Autodesk Inventor part; units mm, degrees
ref_plane "YZ Plane" through (0, 0, 0) normal (1, 0, 0) x (0, 1, 0)
ref_plane "XZ Plane" through (0, 0, 0) normal (0, 1, 0) x (-1, 0, 0)
ref_plane "XY Plane" through (0, 0, 0) normal (0, 0, 1) x (1, 0, 0)
sketch "Sketch1" plane through (0, 0, 0) normal (0, 0, 1) x (1, 0, 0)
  arc A0 (25.4, 0) -> (-25.4, 0.0312) centre (0, 0) ccw
  arc A1 (31.75, 0) -> (-31.75, 0.039) centre (0, 0) ccw
  arc A2 (-31.75, 0.039) -> (-25.4, 0.0312) centre (-28.575, 0.0351) ccw
  line L0 (25.4, 0) -> (25.4, -50.8)
  line L1 (25.4, -50.8) -> (31.75, -50.8)
  line L2 (31.75, -50.8) -> (31.75, 0)
  line L3 (25.4, 0) -> (31.75, 0) construction
  dimension "d0" = 6.35
  dimension "d1" = 25.4
  dimension "d2" = 50.8
extrude "Extrusion1" add sketch "Sketch1" along normal blind 6.35
properties part number "HangHook" material "Steel, High Strength Low Alloy"
Geometry: final body of the model. Coordinates: model frame, mm. Give positions to 0.01 mm unless a question says otherwise; leave off trailing zeros. Loops run counter-clockwise (first coordinate to the right, second up) from the corner with the lowest first, then second, coordinate; pieces in that order, holes last. Notation, with made-up numbers: (-30.5, 45) -> (25.5, 45) arc R35 cw to (25.5, 77) -> close; hole circle Ø11 at (16.5, 75). An arc over 180 degrees is marked (long way). Use one line per item in the form item = value.
Item 1: Draft query along X for faces 1 (the face through (31.75, -26, 3)), 2 (the face through (-0.543, 25.394, 3.131)), 3 (the face through (-0.678, 31.743, 3.131)), 4 (the face through (26, 0, 0)). Return one class per face: pulls with the +X half, pulls with the -X half, needs draft (parallel to the pull), parting line crosses it, or undercut.
A:
face_1 = pulls with the +X half
face_2 = undercut
face_3 = parting line crosses it
face_4 = needs draft
Item 2: Section query B-B on y = -22. Output: boundary loops of the cut face in (x, z).
A:
outline = (25.4, 0) -> (31.75, 0) -> (31.75, 6.35) -> (25.4, 6.35) -> close
Item 3: Section query C-C on z = 4. Output: boundary loops of the cut face in (x, y) (3 decimals), and give its area (3 significant figures).
A:
outline = (-31.75, 0.039) arc R3.175 ccw to (-25.4, 0.031) arc R25.4 cw to (25.4, 0) -> (25.4, -50.8) -> (31.75, -50.8) -> (31.75, 0) arc R31.75 ccw to start
area = 908 mm^2
Item 4: Line query: probe 1 along X at (y, z) = (15, 1.5); probe 2 along X at (y, z) = (-44.5, 1.25); probe 3 along X at (y, z) = (11, 1.5). Output: solid intervals per line, ascending.
A:
probe_1 = -27.98 to -20.5, 20.5 to 27.98
probe_2 = 25.4 to 31.75
probe_3 = -29.78 to -22.89, 22.89 to 29.78
Item 5: Section query D-D on y = 23. Output: boundary loops of the cut face in (x, z).
A:
outline = (-21.89, 0) -> (-10.78, 0) -> (-10.78, 6.35) -> (-21.89, 6.35) -> close; (10.78, 0) -> (21.89, 0) -> (21.89, 6.35) -> (10.78, 6.35) -> close
Item 6: Section query A-A on y = 6. Output: boundary loops of the cut face in (x, z).
A:
outline = (-31.18, 0) -> (-24.68, 0) -> (-24.68, 6.35) -> (-31.18, 6.35) -> close; (24.68, 0) -> (31.18, 0) -> (31.18, 6.35) -> (24.68, 6.35) -> close
Item 7: Pin query (flat end, axial travel): P1, Ø2, axis at x = -13, z = 4.5, coming from the +Y side; P2, Ø12, axis at x = 10, y = 19, coming from the +Z side; P3, Ø1, axis at y = -29, z = 5.5, coming from the -X side. Return the tip coordinate at first contact, or that it passes through.
A:
P1 = 29.39
P2 = 6.35
P3 = 25.4
